Source: three-view drawing plus pictorial views. Frame: mm from the lowest corner of the part. Give positions to 0.01 mm unless a question says otherwise; leave off trailing zeros. Loops run counter-clockwise (first coordinate to the right, second up) from the corner with the lowest first, then second, coordinate; pieces in that order, holes last.
1. Section B-B, the plane y = 1.1. Output: boundary loops of the cut face in (x, z).
2. Section D-D, the plane x = 4. Output: boundary loops of the cut face in (y, z), then the cut area to 3 significant figures.
3. Section C-C, the plane z = 62.5. Output: boundary loops of the cut face in (x, y), then the cut area to 3 significant figures.
4. First-contact query: P1, Ø1.2, axis at y = 2, z = 55.5, coming from the -X side; P2, Ø1.5, axis at x = 5, y = 0.5, coming from the +Z side; P3, Ø1, axis at y = 2, z = 61, coming from the +X side. Flat tips, straight axial feed; report the tip coordinate or a pass-through.
5. Section A-A, the plane z = 7. Output: boundary loops of the cut face in (x, y), then the cut area to 4 significant figures.
6. Material intervals for line 1 along Z through (x, y) = (25, 0.6); line 2 along X through (y, z) = (1.85, 52.5); line 3 along Z through (x, y) = (35, 2.15), sorted ascending.
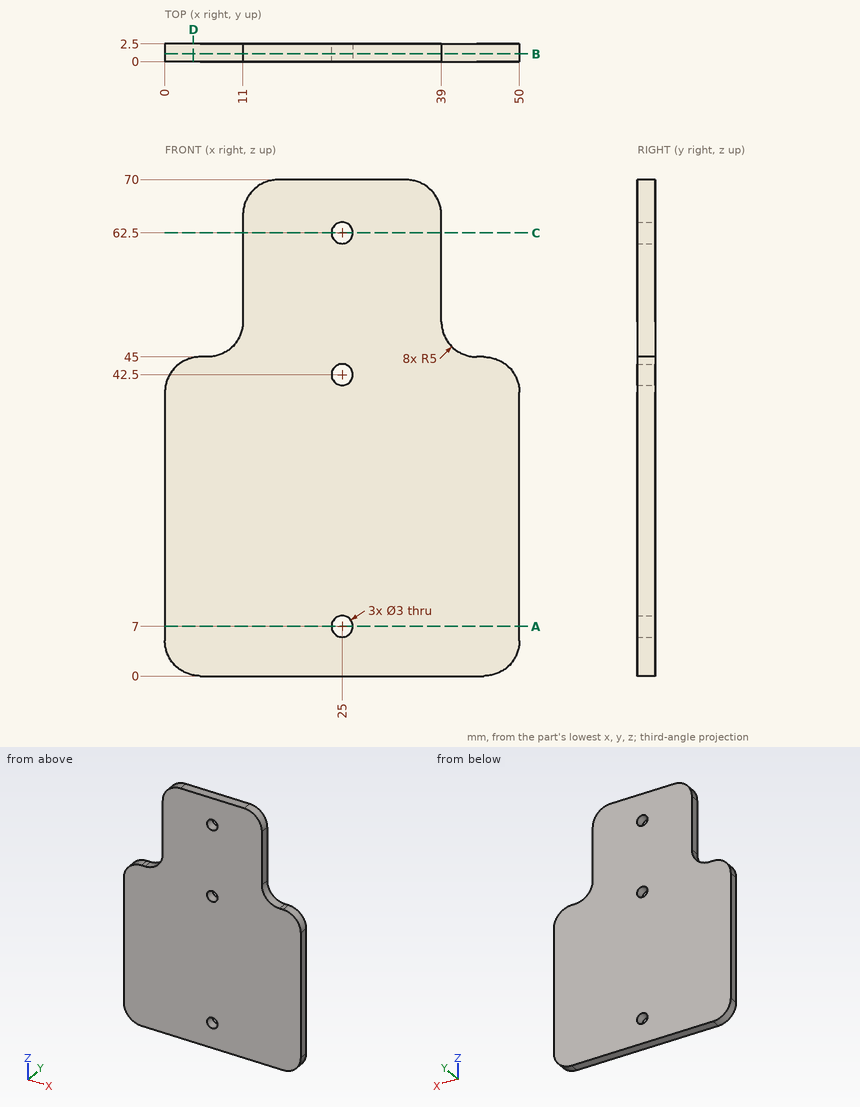
Answers below:
1. outline: (0, 5) arc R5 ccw to (5, 0) - (45, 0) arc R5 ccw to (50, 5) - (50, 40) arc R5 ccw to (45, 45) - (44, 45) arc R5 cw to (39, 50) - (39, 65) arc R5 ccw to (34, 70) - (16, 70) arc R5 ccw to (11, 65) - (11, 50) arc R5 cw to (6, 45) - (5, 45) arc R5 ccw to (0, 40) - close; hole circle Ø3 at (25, 7); hole circle Ø3 at (25, 42.5); hole circle Ø3 at (25, 62.5)
2. outline: (0, 0.1) - (2.5, 0.1) - (2.5, 44.9) - (0, 44.9) - close
2. area: 112 mm2
3. outline: (11, 0) - (23.5, 0) - (23.5, 2.5) - (11, 2.5) - close; (26.5, 0) - (39, 0) - (39, 2.5) - (26.5, 2.5) - close
3. area: 62.5 mm2
4. P1: stops at x = 11
4. P2: stops at z = 45
4. P3: stops at x = 39
5. outline: (0, 0) - (23.5, 0) - (23.5, 2.5) - (0, 2.5) - close; (26.5, 0) - (50, 0) - (50, 2.5) - (26.5, 2.5) - close
5. area: 117.5 mm2
6. line 1: z = 0 to 5.5, 8.5 to 41, 44 to 61, 64 to 70
6. line 2: x = 11 to 39
6. line 3: z = 0 to 69.9
